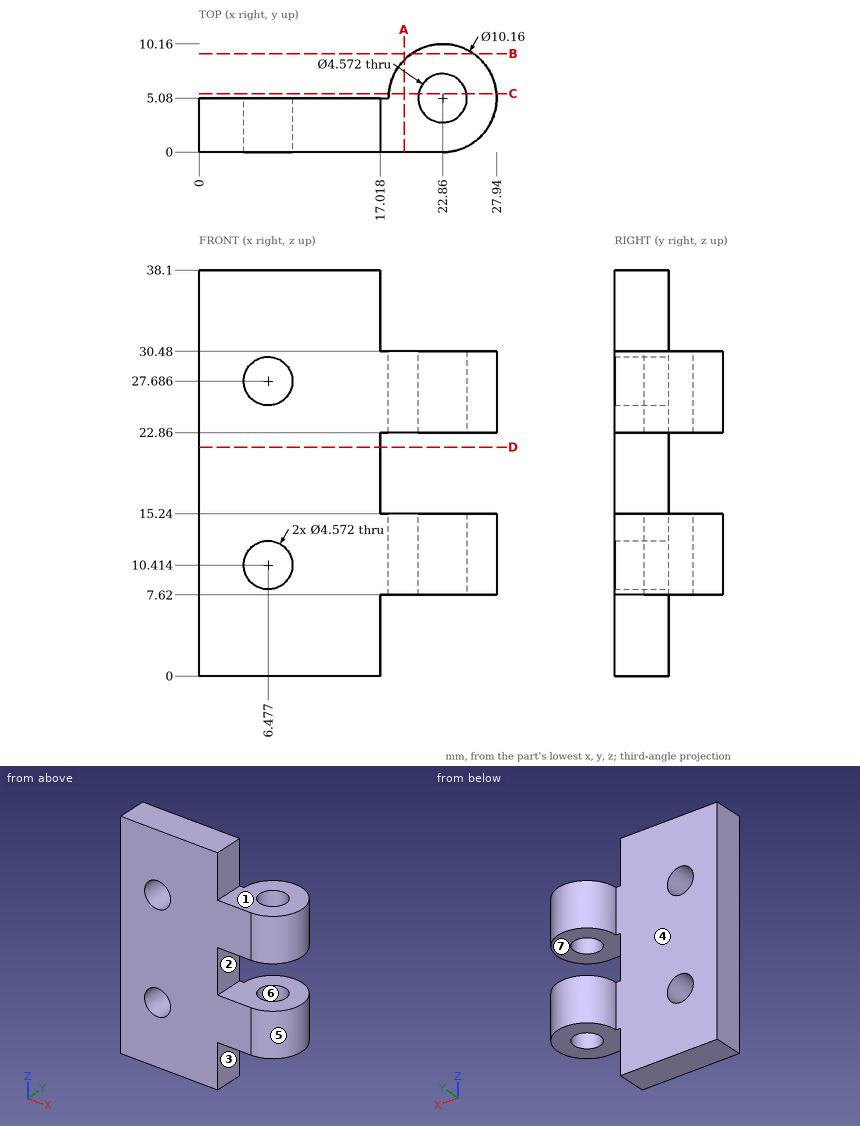
Study the drawing (mm; zero at the part's minimum x, y, z) and answer. A direction names the side the tool comes from. Coordinates: 2 decimals unless noted, no trailing zeros. Loops run counter-clockwise (first coordinate to the right, second up) from the corner with the lowest first, then second, coordinate; pieces in that order, holes last. Notation, with made-up numbers: (-33, 61.5) -> (-6, 61.5) arc R12 cw to (-6, 75.5) -> close; hole circle Ø4 at (87.5, -9.75). An arc over 180 degrees is marked (long way). Answer as CSV lines item,"result".
1) The part is cut by section A-A (x = 19.25). Give the vertices of the cut face in (y, z).
A:
outline,"(0, 7.62) -> (8.65, 7.62) -> (8.65, 15.24) -> (0, 15.24) -> close; (0, 22.86) -> (8.65, 22.86) -> (8.65, 30.48) -> (0, 30.48) -> close"
2) For a pull along Y with two mould halves and no side action, classify the marked faces 5, 6 and 7 as released by +Y, released by -Y, zero draft, split by the parting line, or undercut.
A:
face 5,"split by the parting line"
face 6,"undercut"
face 7,"zero draft"
3) Straight lines are drawn through the part: probe 1 along Z at (x, y) = (24.25, 3); probe 2 along Z at (x, y) = (5.5, 1.5); probe 3 along Z at (x, y) = (7, 3.25). For each, find the intervals that lie inside material, in ascending order.
A:
probe 1,"z = 7.62 to 15.24, 22.86 to 30.48"
probe 2,"z = 0 to 8.35, 12.48 to 25.62, 29.75 to 38.1"
probe 3,"z = 0 to 8.19, 12.64 to 25.46, 29.91 to 38.1"
4) The part is cut by section D-D (z = 21.5). Give the vertices of the cut face in (x, y).
A:
outline,"(0, 0) -> (17.02, 0) -> (17.02, 5.08) -> (0, 5.08) -> close"
5) The part is cut by section C-C (y = 5.5). Give the vertices of the cut face in (x, z).
A:
outline,"(17.8, 7.62) -> (20.61, 7.62) -> (20.61, 15.24) -> (17.8, 15.24) -> close; (17.8, 22.86) -> (20.61, 22.86) -> (20.61, 30.48) -> (17.8, 30.48) -> close; (25.11, 7.62) -> (27.92, 7.62) -> (27.92, 15.24) -> (25.11, 15.24) -> close; (25.11, 22.86) -> (27.92, 22.86) -> (27.92, 30.48) -> (25.11, 30.48) -> close"
6) The part is cut by section B-B (y = 9.25). Give the vertices of the cut face in (x, z).
A:
outline,"(19.96, 7.62) -> (25.76, 7.62) -> (25.76, 15.24) -> (19.96, 15.24) -> close; (19.96, 22.86) -> (25.76, 22.86) -> (25.76, 30.48) -> (19.96, 30.48) -> close"
7) Flat-ended cylindrical pins translate along their axes: pin 1 (1.5 mm diameter, centred on y = 2, z = 18.5, fed in from +X); pin 2 (3.5 mm diameter, centred on x = 22.86, y = 5.08, fed in from +Z); pin 3 (2 mm diameter, centred on x = 13.5, z = 16, fed in from +Y); pin 4 (3 mm diameter, centred on x = 25, y = 2.5, fed in from +Z). Find the tip coordinate at first contact, or state that the pin passes through.
A:
pin 1,"stops at x = 17.02"
pin 2,"passes through"
pin 3,"stops at y = 5.08"
pin 4,"stops at z = 30.48"
8) For the marked faces 1, 2, 3 and 4, determine the directions among +Z, -Z, +X, -X, +Y, -Y from which every point of the face is accessible in a straight line to the end or side of a thin tool.
A:
face 1,"+Z, +X, +Y, -Y"
face 2,"+X, +Y, -Y"
face 3,"-Z, +X, +Y, -Y"
face 4,"+Z, -Z, -X, +Y"
